Can you work these out from the model? Positions are in its coordinate system, mm. A direction names the side the tool comes from. Coordinates: 2 decimals unless noted, no trailing zeros. Loops run counter-clockwise (first coordinate to the right, second up) from the corner with the lowest first, then second, coordinate; pieces in that order, holes last.
Autodesk Fusion 360 part; units mm, degrees
sketch "Sketch1" plane through (0, 0, 0) normal (0, 0, 1) x (1, 0, 0)
  line L0 (185, -95) -> (-185, -95)
  line L1 (-185, -95) -> (-185, 95)
  line L2 (-185, 95) -> (185, 95)
  line L3 (185, 95) -> (185, -95)
  line L4 (185, -95) -> (-185, 95) construction
  line L5 (-185, -95) -> (185, 95) construction
  line L6 (180, -90) -> (-180, -90)
  line L7 (-180, -90) -> (-180, 90)
  line L8 (-180, 90) -> (180, 90)
  line L9 (180, 90) -> (180, -90)
  line L10 (180, -90) -> (-180, 90) construction
  line L11 (-180, -90) -> (180, 90) construction
  line L12 (-185, -95) -> (-200, -95)
  line L13 (-200, -95) -> (-200, -100)
  line L14 (-200, -100) -> (200, -100)
  line L15 (185, -95) -> (200, -95)
  line L16 (200, -95) -> (200, -100)
  dimension "d1" = 370
  dimension "d2" = 190
  dimension "d3" = 360
  dimension "d4" = 180
  dimension "d5" = 400
  dimension "d6" = 15
  dimension "d7" = 5
extrude "Extrude1" add sketch "Sketch1" along normal blind 75 contours L0 L1 L2 L3
extrude "Extrude2" add sketch "Sketch1" along normal blind 5 contours L6 L7 L8 L9
extrude "Extrude3" add sketch "Sketch1" along normal blind 80 and the other way blind 5 contours L0 L12 L13 L14 L15 L16
sketch "Sketch9" plane through (185, 0, 0) normal (1, 0, 0) x (0, 1, 0)
  line L0 (-95, 0) -> (95, 0)
  line L1 (95, 0) -> (95, 75)
  line L2 (95, 75) -> (-95, 75)
  line L3 (-95, 75) -> (-95, 0)
  line L4 (0, 0) -> (0, 60) construction
  line L5 (0, 60) -> (95, 60) construction
  line L6 (0, 60) -> (-95, 60) construction
  line L7 (-95, 60) -> (95, 60)
  line L8 (95, 60) -> (95, 65)
  line L9 (95, 65) -> (-95, 65)
  line L10 (-95, 65) -> (-95, 60)
  dimension "d48" = 5
  dimension "d49" = 60
extrude "Extrude10" add sketch "Sketch9" along normal blind 10 contours L1 L3 L7 L8 L9 L10
sketch "Sketch10" plane through (0, 0, 60) normal (0, 0, -1) x (1, 0, 0)
  line L0 (185, 95) -> (185, -95)
  line L1 (185, -95) -> (195, -95)
  line L2 (195, -95) -> (195, 95)
  line L3 (195, 95) -> (185, 95)
  line L4 (195, -95) -> (190, -95)
  line L5 (190, -95) -> (190, 95)
  line L6 (190, 95) -> (195, 95)
  line L7 (195, 95) -> (195, -95)
extrude "Extrude11" add sketch "Sketch10" along normal blind 5 contours L1 L2 L3 L4 L5 L6 L7
sketch "Sketch11" plane through (-185, 0, 0) normal (-1, 0, 0) x (0, -1, 0)
  line L0 (-95, 0) -> (95, 0)
  line L1 (95, 0) -> (95, 75)
  line L2 (95, 75) -> (-95, 75)
  line L3 (-95, 75) -> (-95, 0)
  line L4 (0, 0) -> (0, 60) construction
  line L5 (95, 60) -> (-95, 60)
  line L6 (-95, 60) -> (-95, 65)
  line L7 (-95, 65) -> (95, 65)
  line L8 (95, 65) -> (95, 60)
  dimension "d54" = 5
  dimension "d55" = 190
  dimension "d56" = 60
extrude "Extrude12" add sketch "Sketch11" along normal blind 10 contours L1 L3 L5 L6 L7 L8
sketch "Sketch13" plane through (0, 0, 60) normal (0, 0, -1) x (1, 0, 0)
  line L0 (-185, -95) -> (-185, 95)
  line L1 (-185, 95) -> (-195, 95)
  line L2 (-195, 95) -> (-195, -95)
  line L3 (-195, -95) -> (-185, -95)
  line L4 (-190, -95) -> (-195, -95)
  line L5 (-195, -95) -> (-195, 95)
  line L6 (-195, 95) -> (-190, 95)
  line L7 (-190, 95) -> (-190, -95)
extrude "Extrude13" add sketch "Sketch13" along normal blind 5 contours L1 L2 L3 L4 L5 L6 L7
sketch "Sketch14" plane through (0, 0, 0) normal (1, 0, 0) x (0, 1, 0)
  curve L0
  line L1 (-100, 80) -> (-114.1421, 65.8579)
  line L2 (-100, 80) -> (-120, 80) construction
  line L3 (-114.1421, 65.8579) -> (-114.1421, 60.8579)
  line L4 (-100, 80) -> (-100, 75)
  line L5 (-100, 75) -> (-114.1421, 60.8579)
  dimension "d61" = 45
  dimension "d62" = 20
  dimension "d63" = 5
extrude "Extrude14" add sketch "Sketch14" along normal mid plane 400
Item 1: I need wall thicknesses on line 1 along X through (y, z) = (75.5, 59); line 2 along X through (y, z) = (68, 10); line 3 along Y through (x, z) = (-63.5, 14). Which ranges of each line are inside material? Lowest first, please.
Results are:
line 1: x = -195 to -190, -185 to -180, 180 to 185, 190 to 195
line 2: x = -185 to -180, 180 to 185
line 3: y = -100 to -90, 90 to 95
Item 2: Suppose I cut it at C-C, the plane y = -58. Please give me the cut outline in (x, z), plus the area to 3 significant figures.
Results are:
outline: (-195, 55) - (-190, 55) - (-190, 60) - (-185, 60) - (-185, 0) - (185, 0) - (185, 60) - (190, 60) - (190, 55) - (195, 55) - (195, 65) - (185, 65) - (185, 75) - (180, 75) - (180, 5) - (-180, 5) - (-180, 75) - (-185, 75) - (-185, 65) - (-195, 65) - close
area: 2,700 mm2
Item 3: On a 3-axis mill with a long thin cutter (end or side, diameter ignored), from which of +Z, -Z, +X, -X, +Y, -Y can I reach the whole of each face in a straight line? I mean faces 1 (the face through (-190, 1, 65)), 2 (the face through (-3, 1, 0)), 3 (the face through (195, 1, 60)). Say none if no direction works.
Results are:
face 1: +Z, -X, +Y
face 2: -Z, +X, -X, +Y
face 3: +Z, -Z, +X, +Y
Item 4: Suppose I cut it at B-B, the plane x = 22. Please give me the cut outline in (y, z), plus the area to 3 significant figures.
Results are:
outline: (-114.14, 60.86) - (-100, 75) - (-100, -5) - (-95, -5) - (-95, 0) - (95, 0) - (95, 75) - (90, 75) - (90, 5) - (-90, 5) - (-90, 75) - (-95, 75) - (-95, 80) - (-100, 80) - (-114.14, 65.86) - close
area: 2,150 mm2
Item 5: Suppose I cut it at A-A, the plane z = 51. Please give me the cut outline in (x, y).
Results are:
outline: (-200, -100) - (200, -100) - (200, -95) - (185, -95) - (185, 95) - (-185, 95) - (-185, -95) - (-200, -95) - close; hole (-180, -90) - (180, -90) - (180, 90) - (-180, 90) - close
Item 6: I'm going to push flat-ended pins straight in: P1, Ø5.5, axis at x = 187, y = 34.5, coming from the -Z side; P2, Ø18, axis at y = -33, z = 30.5, coming from the +X side; P3, Ø5.5, axis at x = -191.5, y = 18, coming from the -Z side. Where does each tip first touch, or does it pass through?
Results are:
P1: stops at z = 0
P2: stops at x = 185
P3: stops at z = 55
Item 7: We'd pull the mould along X, two halves only. Please class faces 4 (the face through (-3, -100, 34)), 5 (the face through (-200, -99, 44)), 6 (the face through (185, 1, 70)), 7 (the face through (3, -90, 40)): +X half, -X half, draft (parallel to the pull), parting line (faces both ways), or undercut.
Results are:
face 4: draft
face 5: -X half
face 6: +X half
face 7: undercut
